Model file for the job. Use its own axes, mm. Face numbers are marked on the shaded views. A direction names the side the tool comes from. Coordinates: 2 decimals unless noted, no trailing zeros. Order: outer loops, then holes, each group sorted by start corner. A loop starts at its lowest first (then second) coordinate and runs counter-clockwise, first axis right, second up.
from build123d import *

# Parameters (mm, degrees)
SKETCH2_R           = 2.44
BOSS_EXTRUDE1_DEPTH = 1.5
SKETCH3_R           = 3.1
BOSS_EXTRUDE2_DEPTH = 3.5
SKETCH4_R           = 2.665
BOSS_EXTRUDE3_DEPTH = 0.87


with BuildPart() as part:
    # Sketch1 → Revolve1 (revolve)
    with BuildSketch(Plane(origin=(0, 0, 0), x_dir=(1, 0, 0), z_dir=(0, 1, 0))):
        with BuildLine():
            Line((0, 0), (0, -6))
            Line((0, -6), (20.3, -6))
            add(Edge.make_bspline(
                [(20.3, -6), (29.637498304, -5.936932341), (42.015719343, -5.941972282), (53.939810571, -3.018068917), (57.010038962, -1.04718188), (57.201526924, -0.070177055), (57.2, 0)],
                knots=[0, 0, 0, 0, 0.74911683, 0.92248095, 0.994604009, 1, 1, 1, 1], degree=3))
            Line((57.2, 0), (0, 0))
        make_face()
    revolve(axis=Axis((0, 0, 0), (1, 0, 0)))

    # Sketch2 → Boss-Extrude1 (add)
    with BuildSketch(Plane.ZY):
        Circle(SKETCH2_R)
    extrude(amount=BOSS_EXTRUDE1_DEPTH)

    # Sketch3 → Boss-Extrude2 (add)
    with BuildSketch(Plane.ZY.offset(1.5)):
        Circle(SKETCH3_R)
    extrude(amount=BOSS_EXTRUDE2_DEPTH)

    # Sketch4 → Boss-Extrude3 (add)
    with BuildSketch(Plane.ZY.offset(5)):
        Circle(SKETCH4_R)
    extrude(amount=BOSS_EXTRUDE3_DEPTH)


solid = part.part
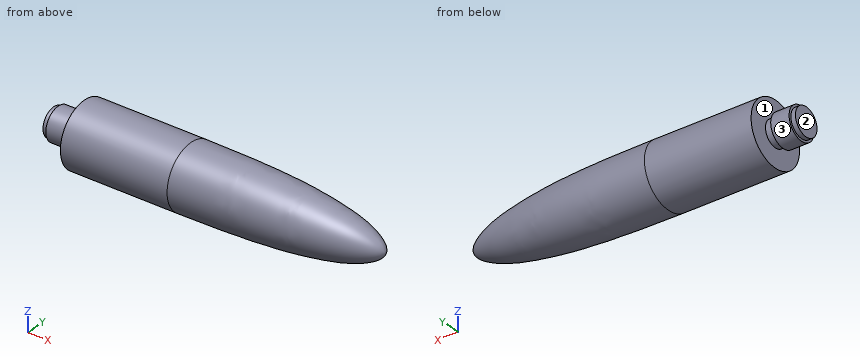
Q1. Probe line 1 (Y direction, x = 20.5, z = 0); line 2 (X direction, y = -2.5, z = 0.5); line 3 (X direction, y = -2.5, z = 0.25). List the from-to ranges inside material, lowest first.
Established:
line 1: y = -6 to 6
line 2: x = -5.87 to -1.5, 0 to 54.3
line 3: x = -5.87 to -1.5, 0 to 54.39
Q2. Drop flat-ended pins along their axis: P1, Ø6, axis at y = 3.5, z = 2, coming from the +X side; P2, Ø2, axis at x = 41, z = 2, coming from the -Y side; P3, Ø2, axis at x = 18.5, y = -2.5, coming from the +Z side. Give the stop position or say it passes through.
Established:
P1: stops at x = 56.72
P2: stops at y = -5.2
P3: stops at z = 5.81
Q3. Cut at A-A, the plane x = 2.5. List the corners of the cut face in (y, z), plus the area to 3 significant figures.
Established:
outline: circle Ø12 at (0, 0)
area: 113 mm2
Q4. Which spindle directions (+Z, -Z, +X, -X, +Y, -Y) get a long thin tool onto all of the face, cutting with end or side? Do the marked faces 1, 2 and 3. Say none if no direction does.
Established:
face 1: none
face 2: +Z, -Z, -X, +Y, -Y
face 3: -X
